Input: part model. Units: mm. Frame: model coordinates. Face numbers are marked on the shaded views. Round coordinates to 2 decimals unless told otherwise and drop trailing zeros. Loops run counter-clockwise (first coordinate to the right, second up) from the corner with the lowest first, then second, coordinate; pieces in that order, holes last. Notation, with made-up numbers: M -37,72.25 L -1,72.25 A25 ccw -1,98.25 Z; hole C -5.5,52.25 d5. An arc over 180 degrees is marked long. Use one line per item in the form item = value. Start each with the question number.
Q1. Ray query, line 1 along Z through (x, y) = (44.5, 25.75); line 2 along Y through (x, z) = (26, -13.25); line 3 along Y through (x, z) = (22.5, -5.5) (3 decimals). Return the intervals inside material, ascending.
Q2. Section query A-A, the plane y = -18. Output: boundary loops of the cut face in (x, z) (3 decimals), and give its area (3 significant figures).
Q3. Section query C-C, the plane y = -7.5. Output: boundary loops of the cut face in (x, z).
Q4. Mould query, pull axis Z, two halves, no side actions, for the marked faces 1, 2 and 3. Classes: pulls with the +Z half, pulls with the -Z half, needs draft (parallel to the pull), parting line crosses it, or undercut.
Q5. Section query B-B, the plane z = 5.5. Output: boundary loops of the cut face in (x, y) (3 decimals).
Q6. First-contact query: P1, Ø3.5, axis at y = 18, z = -13.25, coming from the -X side; P2, Ø4, axis at x = 22, y = 9, coming from the -Z side; P3, Ø1.5, axis at x = 23, z = -16, coming from the +Y side; P4, Ø10, axis at x = 66, y = -6.5, coming from the +Z side. Flat tips, straight axial feed; report the tip coordinate or a pass-through.
```python
from build123d import *

# Parameters (mm, degrees)
EXTRUDE_1_DEPTH             = 90
SKETCH_2_W                  = 90
SKETCH_2_H                  = 17.75
EXTRUDE_2_DEPTH             = 8.2
SKETCH_3_W                  = 90
SKETCH_3_H                  = 50.95
EXTRUDE_3_DEPTH             = 8.2
SKETCH_4_W                  = 3.95
SKETCH_4_H                  = 29.5
CUT_EXTRUDE_1_DEPTH         = 91
SKETCH_5_W                  = 3.95
SKETCH_5_H                  = 6.2
CUT_EXTRUDE_2_DEPTH         = 91
SKETCH_6_W                  = 2.25
SKETCH_6_H                  = 3.95
CUT_EXTRUDE_3_DEPTH         = 91
SKETCH_7_W                  = 4.5
SKETCH_7_H                  = 3.95
CUT_EXTRUDE_4_DEPTH         = 91
SKETCH_8_W                  = 2.25
SKETCH_8_H                  = 3.95
CUT_EXTRUDE_5_DEPTH         = 91
SKETCH_9_W                  = 3.95
SKETCH_9_H                  = 2.25
CUT_EXTRUDE_6_DEPTH         = 91
SKETCH_10_W                 = 19.6
SKETCH_10_H                 = 44.6
CUT_EXTRUDE_7_DEPTH         = 86.2
HOLE_WIZARD_2_5_2_5_1_D     = 2.5
HOLE_WIZARD_2_5_2_5_1_DEPTH = 90
HOLE_WIZARD_4_5_4_5_1_D     = 4.5
HOLE_WIZARD_4_5_4_5_1_DEPTH = 90
FILLET_1_R                  = 2
FILLET_2_R                  = 2
SKETCH_17_R                 = 1.25
EXTRUDE_4_DEPTH             = 90
EXTRUDE_5_DEPTH             = 0.2


with BuildPart() as part:
    # Эскиз1 → Бобышка-Вытянуть1 (new body)
    with BuildSketch(Plane(origin=(90, 0, 0), x_dir=(0, 0, -1), z_dir=(1, 0, 0))):
        with BuildLine():
            Line((6.75, -24.093761792), (6.75, 19.25))
            Line((6.75, 19.25), (-11.593761792, 19.25))
            ThreePointArc((-11.593761792, 19.25), (-15.325, 18), (-11.593761792, 16.75))
            Line((-11.593761792, 16.75), (-11, 16.75))
            Line((-11, 16.75), (-11, -16.75))
            Line((-11, -16.75), (-11.593761792, -16.75))
            ThreePointArc((-11.593761792, -16.75), (-15.325, -18), (-11.593761792, -19.25))
            Line((-11.593761792, -19.25), (-11, -19.25))
            Line((-11, -19.25), (-11, -23.5))
            Line((-11, -23.5), (-6.75, -23.5))
            Line((-6.75, -23.5), (-6.75, -24.093761792))
            ThreePointArc((-6.75, -24.093761792), (-5.5, -27.825), (-4.25, -24.093761792))
            Line((-4.25, -24.093761792), (-4.25, -23.5))
            Line((-4.25, -23.5), (4.25, -23.5))
            Line((4.25, -23.5), (4.25, -24.093761792))
            ThreePointArc((4.25, -24.093761792), (5.5, -27.825), (6.75, -24.093761792))
        make_face()
    extrude(amount=-EXTRUDE_1_DEPTH)

    # Эскиз2 → Бобышка-Вытянуть2 (add)
    with BuildSketch(Plane(origin=(0, 19.25, 0), x_dir=(-1, 0, 0), z_dir=(0, 1, 0))):
        with Locations((-45, 2.125)):
            Rectangle(SKETCH_2_W, SKETCH_2_H)
    extrude(amount=EXTRUDE_2_DEPTH)

    # Эскиз3 → Бобышка-Вытянуть3 (add)
    with BuildSketch(Plane(origin=(0, 0, -6.75), x_dir=(-1, 0, 0), z_dir=(0, 0, -1))):
        with Locations((-45, 1.975)):
            Rectangle(SKETCH_3_W, SKETCH_3_H)
    extrude(amount=EXTRUDE_3_DEPTH)

    # Эскиз4 → Вырез-Вытянуть1 (cut, through all)
    with BuildSketch(Plane.ZY):
        with Locations((-12.975, 0)):
            Rectangle(SKETCH_4_W, SKETCH_4_H)
    extrude(amount=-CUT_EXTRUDE_1_DEPTH, mode=Mode.SUBTRACT)

    # Эскиз5 → Вырез-Вытянуть2 (cut, through all)
    with BuildSketch(Plane.ZY):
        with Locations((-12.975, 24.35)):
            Rectangle(SKETCH_5_W, SKETCH_5_H)
    extrude(amount=-CUT_EXTRUDE_2_DEPTH, mode=Mode.SUBTRACT)

    # Эскиз6 → Вырез-Вытянуть3 (cut, through all)
    with BuildSketch(Plane.ZY):
        with Locations((-9.875, 25.475)):
            Rectangle(SKETCH_6_W, SKETCH_6_H)
    extrude(amount=-CUT_EXTRUDE_3_DEPTH, mode=Mode.SUBTRACT)

    # Эскиз7 → Вырез-Вытянуть4 (cut, through all)
    with BuildSketch(Plane.ZY):
        with Locations((0, 25.475)):
            Rectangle(SKETCH_7_W, SKETCH_7_H)
    extrude(amount=-CUT_EXTRUDE_4_DEPTH, mode=Mode.SUBTRACT)

    # Эскиз8 → Вырез-Вытянуть5 (cut, through all)
    with BuildSketch(Plane.ZY):
        with Locations((9.875, 25.475)):
            Rectangle(SKETCH_8_W, SKETCH_8_H)
    extrude(amount=-CUT_EXTRUDE_5_DEPTH, mode=Mode.SUBTRACT)

    # Эскиз9 → Вырез-Вытянуть6 (cut, through all)
    with BuildSketch(Plane.ZY):
        with Locations((-12.975, -22.375)):
            Rectangle(SKETCH_9_W, SKETCH_9_H)
    extrude(amount=-CUT_EXTRUDE_6_DEPTH, mode=Mode.SUBTRACT)

    # Эскиз10 → Вырез-Вытянуть7 (cut)
    with BuildSketch(Plane(origin=(90, 0, 0), x_dir=(0, 0, -1), z_dir=(1, 0, 0))):
        Rectangle(SKETCH_10_W, SKETCH_10_H)
    extrude(amount=-CUT_EXTRUDE_7_DEPTH, mode=Mode.SUBTRACT)

    # Диаметр отверстия Ø2.5 (2.5)1
    with Locations(Plane(origin=(90, 0, 0), x_dir=(0, 0, -1), z_dir=(1, 0, 0))):
        with Locations((5.5, -25.75), (-13.25, -18), (-5.5, -25.75), (-13.25, 18)):
            Hole(HOLE_WIZARD_2_5_2_5_1_D / 2, depth=HOLE_WIZARD_2_5_2_5_1_DEPTH)

    # Диаметр отверстия Ø4.5 (4.5)1
    with Locations(Plane.ZY):
        with Locations((-13.25, -18), (-13.25, 18), (-5.5, 25.75), (5.5, 25.75)):
            Hole(HOLE_WIZARD_4_5_4_5_1_D / 2, depth=HOLE_WIZARD_4_5_4_5_1_DEPTH)

    # Скругление1
    fillet_1_edges = [part.edges().sort_by_distance(p)[0] for p in [
        (45, 23.5, 8.75),
    ]]
    fillet(fillet_1_edges, radius=FILLET_1_R)

    # Скругление2
    fillet_2_edges = [part.edges().sort_by_distance(p)[0] for p in [
        (45, 23.5, -8.75),
        (45, 23.5, 2.25),
        (45, 23.5, -2.25),
        (45, -21.25, -11),
        (45, 14.75, -11),
        (45, -14.75, -11),
        (45, 21.25, -11),
    ]]
    fillet(fillet_2_edges, radius=FILLET_2_R)

    # Эскиз17 → Бобышка-Вытянуть4 (add)
    with BuildSketch(Plane(origin=(90, 0, 0), x_dir=(0, 0, -1), z_dir=(1, 0, 0))):
        with Locations((5.5, -25.75)):
            Circle(SKETCH_17_R)
        with Locations((-5.5, -25.75)):
            Circle(SKETCH_17_R)
        with Locations((-13.25, -18)):
            Circle(SKETCH_17_R)
        with Locations((-13.25, 18)):
            Circle(SKETCH_17_R)
    extrude(amount=-EXTRUDE_4_DEPTH)

    # Эскиз19 → Бобышка-Вытянуть5 (add)
    with BuildSketch(Plane.ZY):
        with BuildLine():
            Line((-14.95, 15.638029851), (-3.138029851, 27.45))
            ThreePointArc((-3.138029851, 27.45), (-17.517080976, 30.017080976), (-14.95, 15.638029851))
        make_face()
        with BuildLine():
            Line((15.325, 18), (3.138029851, 27.45))
            ThreePointArc((3.138029851, 27.45), (15.439952139, 30.731564972), (15.325, 18))
        make_face()
        with BuildLine():
            Line((14.608219689, -16.431285789), (4.121265041, -27.300714324))
            ThreePointArc((4.121265041, -27.300714324), (17.021902806, -29.253720028), (14.608219689, -16.431285789))
        make_face()
        with BuildLine():
            Line((-5.5, -27.825), (-14.95, -15.638029851))
            ThreePointArc((-14.95, -15.638029851), (-18.231564972, -27.939952139), (-5.5, -27.825))
        make_face()
    extrude(amount=-EXTRUDE_5_DEPTH)


solid = part.part
```
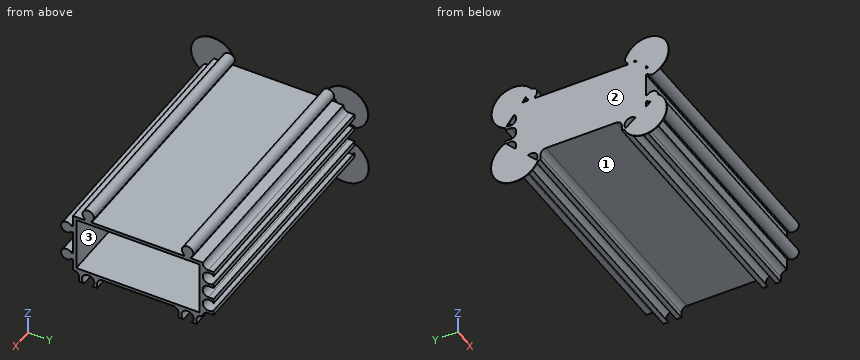
Results found:
q1.line_1 = -8.75 to -7.75, -3.25 to -2.25, 2.25 to 3.25, 7.75 to 8.75
q1.line_2 = -21.25 to -20.25, -15.75 to -14.75, 14.75 to 15.75, 20.25 to 21.25
q1.line_3 = -27.825 to -22.3, 22.3 to 23.5
q2.outline = M 0,-18.124 L 0.2,-18.124 L 0.2,-13.118 L 0,-13.118 Z; M 0,-11 L 90,-11 L 90,-9.8 L 3.8,-9.8 L 3.8,9.8 L 90,9.8 L 90,15.325 L 0.2,15.325 L 0.2,16.879 L 0,16.879 Z
q2.area = 681 mm²
q3.outline = M 0,-11 L 90,-11 L 90,-9.8 L 3.8,-9.8 L 3.8,9.8 L 90,9.8 L 90,11 L 0,11 Z
q4.face_1 = pulls with the -Z half
q4.face_2 = needs draft
q4.face_3 = undercut
q5.outline = M 0,-29.246 L 0.2,-29.246 L 0.2,-27.825 L 90,-27.825 L 90,-22.3 L 3.8,-22.3 L 3.8,22.3 L 90,22.3 L 90,23.5 L 0,23.5 Z; M 0,25.618 L 0.2,25.618 L 0.2,30.624 L 0,30.624 Z
q6.P1 = 0
q6.P2 = -11
q6.P3 = through
q6.P4 = 11
